Autodesk Inventor part; units mm, degrees
ref_plane "Płaszczyzna konstrukcyjna1" through (0, 20, 0) normal (0, 1, 0) x (1, 0, 0)
ref_plane "YZ Plane" through (0, 0, 0) normal (1, 0, 0) x (0, 1, 0)
ref_plane "XZ Plane" through (0, 0, 0) normal (0, 1, 0) x (-1, 0, 0)
sketch "Szkic1" plane through (0, 0, 0) normal (0, 1, 0) x (-1, 0, 0)
  line L0 (-4, -50.1202) -> (-4, -37.2024)
  line L1 (-42.5, -51.8732) -> (-42.5, -51.3513)
  line L2 (-4, -38) -> (-4, -50.1202)
  arc A0 (-38.9822, -45.8888) -> (-34, -38.0004) centre (-42.4987, -38.1503) ccw
  line L3 (-42.5, -51.3513) -> (-42.5, -51.8732)
  arc A1 (-34, -38.0004) -> (-34.0517, -37.2023) centre (-42.4987, -38.1503) ccw
  arc A2 (-38.9822, -45.8888) -> (-42.5, -51.3513) centre (-36.5, -51.3513) ccw
  arc A3 (-42.5, -51.8732) -> (-6.8354, -58.8964) centre (-23.0549, -47.1948) ccw
  arc A4 (-6.8354, -58.8964) -> (-4, -50.1202) centre (-19, -50.1202) ccw
  line L4 (-42.5, -51.3513) -> (-42.5, -51.8732)
  line L5 (-4, -24.2847) -> (-4, -37.2024)
  line L6 (-42.5, -22.5011) -> (-42.5, -23.0533)
  line L7 (-4, -36.4049) -> (-4, -24.2847)
  arc A5 (-34, -36.4047) -> (-38.9822, -28.5157) centre (-42.4987, -36.2542) ccw
  line L8 (-42.5, -23.0533) -> (-42.5, -22.5011)
  arc A6 (-34.0517, -37.2023) -> (-34, -36.4047) centre (-42.4987, -36.2542) ccw
  arc A7 (-42.5, -23.0533) -> (-38.9822, -28.5157) centre (-36.5, -23.0533) ccw
  arc A8 (-6.8187, -15.5316) -> (-42.5, -22.5011) centre (-23.0604, -27.2024) ccw
  arc A9 (-4, -24.2847) -> (-6.8187, -15.5316) centre (-19, -24.2847) ccw
  line L9 (-42.5, -23.0533) -> (-42.5, -22.5011)
  line L10 (-12, -10.5391) -> (-12, -12.5391)
  line L11 (-34.5, -10.7971) -> (-34.5, -12.7971)
  arc A10 (-12, -12.5391) -> (-34.5, -12.7971) centre (-23.0889, -26.7178) ccw
  line L12 (-11.9997, -63.8616) -> (-11.9997, -61.8657)
  line L13 (-34.5004, -63.596) -> (-34.5004, -61.6077)
  arc A11 (-34.5004, -61.6077) -> (-11.9997, -61.8657) centre (-23.0889, -47.6872) ccw
  line L14 (-35.8952, -43.5023) -> (-33.8952, -43.5023)
  line L15 (-35.8952, -30.9023) -> (-33.8952, -30.9023)
  arc A12 (-33.8952, -43.5023) -> (-33.8952, -30.9023) centre (-44.1084, -37.2023) ccw
  line L16 (-4, -28) -> (-6, -28)
  line L17 (-6, -46) -> (-4, -46)
  arc A13 (-6, -46) -> (-6, -28) centre (-89.405, -37) ccw
  line L18 (-40.8175, -18) -> (-38.8175, -18)
  line L19 (-40.8176, -27.2196) -> (-38.8176, -27.2198)
  arc A14 (-38.8175, -18) -> (-38.9822, -27.2198) centre (-34.316, -22.6918) ccw
  line L20 (-41.0122, -56.0002) -> (-39.0216, -56.0002)
  line L21 (-39.0216, -56.0002) -> (-41.0122, -56.0002)
  line L22 (-41.0216, -47.4073) -> (-39.0216, -47.4076)
  arc A15 (-39.0216, -47.4076) -> (-39.0216, -56.0002) centre (-35.5308, -51.7039) ccw
  line L23 (-19, -7.6189) -> (11, -7.6189) construction
  point P0 (0, 0)
  point P1 (-42.5001, -29.6503)
  point P2 (-4, -22.2491)
  point P3 (-23.0549, -67.1948)
  point P4 (-23.0549, -67.1948)
  point P5 (-42.5, -44.7542)
  point P6 (-23.0604, -7.2024)
  point P7 (-23.0604, -7.2024)
  dimension "d12" = 15
  dimension "d13" = 30
  dimension "d14" = 6
  dimension "d15" = 20
  dimension "d21" = 38.5
  dimension "d53" = 2
extrude "Wyciągnięcie proste1" add sketch "Szkic1" along normal blind 5
extrude "Wyciągnięcie proste2" add sketch "Szkic1" against normal blind 2 contours L17 A13 L16 L5 L0 | A3 L13 A11 L12 | A3 L1 A2 L22 A15 L20 | L10 A10 L11 A8 | L18 A14 L19 A7 L6 A8 | A0 A1 A6 A5 L15 A12 L14
sketch "Szkic5" plane through (0, 5, 0) normal (0, 1, 0) x (1, 0, 0)
  line L0 (4, 28) -> (6, 28)
  arc A0 (6, 46) -> (6, 28) centre (89.405, 37) ccw
  line L1 (6, 46) -> (4, 46)
  line L2 (4, 50.1202) -> (4, 46)
  arc A1 (6.8354, 58.8964) -> (4, 50.1202) centre (19, 50.1202) ccw
  arc A2 (11.9997, 63.8616) -> (6.8354, 58.8964) centre (23.0549, 47.1948) ccw
  line L3 (11.9997, 63.8616) -> (11.9997, 61.8657)
  arc A3 (34.5004, 61.6077) -> (11.9997, 61.8657) centre (23.0889, 47.6872) ccw
  line L4 (34.5004, 61.6077) -> (34.5004, 63.596)
  arc A4 (41.0122, 56.0002) -> (34.5004, 63.596) centre (23.0549, 47.1948) ccw
  line L5 (41.0122, 56.0002) -> (39.0216, 56.0002)
  arc A5 (39.0216, 47.4076) -> (39.0216, 56.0002) centre (35.5308, 51.7039) ccw
  line L6 (39.0216, 47.4076) -> (41.0216, 47.4073)
  arc A6 (38.9822, 45.8888) -> (41.0216, 47.4073) centre (36.5, 51.3513) ccw
  arc A7 (38.9822, 45.8888) -> (35.8952, 43.5023) centre (42.4987, 38.1503) ccw
  line L7 (35.8952, 43.5023) -> (33.8952, 43.5023)
  arc A8 (33.8952, 43.5023) -> (33.8952, 30.9023) centre (44.1084, 37.2023) ccw
  line L8 (33.8952, 30.9023) -> (35.8952, 30.9023)
  arc A9 (35.8952, 30.9023) -> (38.9822, 28.5157) centre (42.4987, 36.2542) ccw
  arc A10 (40.8176, 27.2196) -> (38.9822, 28.5157) centre (36.5, 23.0533) ccw
  line L9 (40.8176, 27.2196) -> (38.9822, 27.2198)
  arc A11 (38.8175, 18) -> (38.9822, 27.2198) centre (34.316, 22.6918) ccw
  line L10 (38.8175, 18) -> (40.8175, 18)
  arc A12 (34.5, 10.7971) -> (40.8175, 18) centre (23.0604, 27.2024) ccw
  line L11 (34.5, 10.7971) -> (34.5, 12.7971)
  arc A13 (12, 12.5391) -> (34.5, 12.7971) centre (23.0889, 26.7178) ccw
  line L12 (12, 12.5391) -> (12, 10.5391)
  arc A14 (6.8187, 15.5316) -> (12, 10.5391) centre (23.0604, 27.2024) ccw
  arc A15 (4, 24.2847) -> (6.8187, 15.5316) centre (19, 24.2847) ccw
  line L13 (4, 28) -> (4, 24.2847)
  arc A16 (12, 10.5391) -> (34.5, 10.7971) centre (23.0604, 27.2024) ccw
  arc A17 (34.5004, 63.596) -> (11.9997, 63.8616) centre (23.0549, 47.1948) ccw
  line L14 (4, 28) -> (4, 46)
  arc A18 (40.8175, 18) -> (42.5, 22.5011) centre (23.0604, 27.2024) ccw
  arc A19 (42.5, 23.0533) -> (40.8176, 27.2196) centre (36.5, 23.0533) ccw
  line L15 (42.5, 23.0533) -> (42.5, 22.5011)
  arc A20 (34.0517, 37.2023) -> (35.8952, 30.9023) centre (42.4987, 36.2542) ccw
  arc A21 (35.8952, 43.5023) -> (34.0517, 37.2023) centre (42.4987, 38.1503) ccw
  arc A22 (42.5, 51.8732) -> (41.0122, 56.0002) centre (23.0549, 47.1948) ccw
  line L16 (42.5, 51.8732) -> (42.5, 51.3513)
  arc A23 (41.0216, 47.4073) -> (42.5, 51.3513) centre (36.5, 51.3513) ccw
  arc A24 (6.8187, 15.5316) -> (42.5, 22.5011) centre (23.0604, 27.2024) ccw
  line L17 (20.4612, 7.372) -> (50.4612, 7.372) construction
  line L18 (4, 50.1202) -> (4, 24.2847)
  circle A25 centre (19, 37.372) radius 10
  dimension "d74" = 20
ref_plane "Płaszczyzna konstrukcyjna1" through (0, 20, 0) normal (0, 1, 0) x (1, 0, 0)
sketch "Szkic6" plane through (0, 20, 0) normal (0, 1, 0) x (1, 0, 0)
  circle A0 centre (19, 37.372) radius 5
  point P0 (0, 0)
  dimension "d76" = 10
loft "Wyciągnięcie złożone1" add profiles "Szkic6", "Szkic5" contours all / A25
sketch "Szkic7" plane through (19, 20, -37.372) normal (0, 1, 0) x (1, 0, 0)
  circle A0 centre (0, 0) radius 5
  point P0 (-19, -37.372)
  dimension "d85" = 10
extrude "Wyciągnięcie proste3" add sketch "Szkic7" along normal blind 15
fillet "Zaokrąglenie1" radius 5 1 edges at (14, 35, -37.372)
properties part number "1" material "Tytan 6Al-4V"
Geometry: final body of the model. Coordinates: model frame, mm. A direction names the side the tool comes from. Give positions to 0.01 mm unless a question says otherwise; leave off trailing zeros. Order: outer loops, then holes, each group sorted by start corner. A loop starts at its lowest first (then second) coordinate and runs counter-clockwise, first axis right, second up. Notation, with made-up numbers: M -3.75,40 L 22.25,40 A20 ccw 22.25,62 Z; hole C -23,-38 d10. An arc over 180 degrees is marked long. Answer as CSV lines item,"result". Start each with the question number.
1) Cut plane B-B (x = 37.5). Output: boundary loops of the cut face in (y, z).
2) Cut plane D-D (z = -26). Output: boundary loops of the cut face in (x, y).
3) Line query: line 1 (Y direction, x = 21, z = -10); line 2 (Z direction, x = 14.5, y = 16.5); line 3 (X direction, y = 8, z = -36.5). Output: solid intervals per line, ascending. Write a range as from..to.
4) Cut plane C-C (x = 19). Output: boundary loops of the cut face in (y, z), then the cut area to 3 significant figures.
5) Cut plane A-A (y = 2). Output: boundary loops of the cut face in (x, z).
6) Mould query, pull axis Z, two halves, no side actions, for faces 1 (the flat face through (5, -1, -28)), 2 (the cylindrical face through (17.916, 24.93, -42.253)), 3 (the flat face through (34.5, -1, -12)), 4 (the flat face through (23, 0, -37)). Classes: +Z half, -Z half, draft (parallel to the pull), parting line (faces both ways), or undercut.
7) First-contact query: P1, Ø2, axis at x = 39.5, y = -0.5, coming from the +Z side; P2, Ø8, axis at x = 18, y = 31, coming from the -Z side; P3, Ø18.5, axis at x = 24, z = -36.5, coming from the -Y side; P4, Ø8, axis at y = 3, z = -17, coming from the -X side. Flat tips, straight axial feed; report the tip coordinate or a pass-through.
8) Set-up query: faces 5 (the flat face through (12, -1, -63)), 6 (the cylindrical face through (5.516, -0.986, -37.126)), 7 (the cylindrical face through (35.349, 2.229, -31.657)). Return all of +Z, -Z, +X, -X, +Y, -Y with unobstructed straight access to the full face (end or side cutting, diameter ignored); none if empty.
Findings below:
1,outline,"M 0,-61.03 L 5,-61.03 L 5,-45.03 L 0,-45.03 Z; M 0,-29.38 L 5,-29.38 L 5,-13.36 L 0,-13.36 Z"
2,outline,"M 4,0 L 39.91,0 L 39.91,-2 L 41.73,-2 L 41.73,5 L 4,5 Z"
3,line 1,"y = 0..5"
3,line 2,"z = -41.59..-33.16"
3,line 3,"x = 10.04..27.96"
4,outline,"M -2,-66.78 L 5,-66.78 L 5,-47.37 L 20,-42.37 L 30,-42.37 A5 ccw 30,-32.37 L 20,-32.37 L 5,-27.37 L 5,-7.62 L -2,-7.62 L -2,-9.19 L 0,-9.19 L 0,-65.22 L -2,-65.22 Z"
4,area,"666 mm²"
5,outline,"M 4,-50.12 A15 ccw 6.84,-58.9 A20 ccw 42.5,-51.87 L 42.5,-51.35 A6 ccw 38.98,-45.89 A8.5 cw 34,-38 A8.5 cw 34.05,-37.2 A8.5 cw 34,-36.4 A8.5 cw 38.98,-28.52 A6 ccw 42.5,-23.05 L 42.5,-22.5 A20 ccw 6.82,-15.53 A15 ccw 4,-24.28 Z"
6,face 1,"+Z half"
6,face 2,"parting line"
6,face 3,"draft"
6,face 4,"undercut"
7,P1,"stops at z = -14.65"
7,P2,"stops at z = -42.37"
7,P3,"stops at y = -2"
7,P4,"stops at x = 4.36"
8,face 5,"+Z, -Z, -X, -Y"
8,face 6,"-Y"
8,face 7,"+X, +Y, -Y"
